Input: part model. Units: mm. Frame: model coordinates. Round coordinates to 2 decimals unless told otherwise and drop trailing zeros. Order: outer loops, then holes, each group sorted by start corner. A loop starts at its lowest first (then second) coordinate and runs counter-clockwise, first axis right, second up.
Item 1: Cut plane B-B on x = -10. Output: boundary loops of the cut face in (y, z).
Item 2: Line query: L1, parallel to Y at x = 0, z = -18.5; L2, parallel to Z at x = 2, y = -429.5 (3 decimals); L3, parallel to X at y = -786, z = 0.5. Output: solid intervals per line, ascending.
Item 3: Cut plane A-A on z = 0. Output: boundary loops of the cut face in (x, y), then the cut area to 3 significant figures.
Item 4: Cut plane C-C on y = -773. Output: boundary loops of the cut face in (x, z), then the cut area to 3 significant figures.
Item 5: First-contact query: pin 1 (5 mm diameter, centred on y = -100.5, z = -13.5, fed in from +X); pin 2 (6 mm diameter, centred on y = -367, z = 3.5, fed in from -X); pin 3 (4 mm diameter, centred on x = 11.5, y = -325.5, fed in from +Z). Flat tips, straight axial feed; report the tip coordinate or a pass-through.
```python
from build123d import *

# Parameters (mm, degrees)
F0_R     = 19.05
F0_R_2   = 17.45
F1_DEPTH = 825
F2_R     = 3.5625283299
F3_DEPTH = 20.050000094
F4_R     = 1
F5_DEPTH = 20.050000107


with BuildPart() as f1:
    # F0 (on Front) → F1 (new body)
    with BuildSketch(Plane.XZ):
        Circle(F0_R)
        Circle(F0_R_2, mode=Mode.SUBTRACT)
    extrude(amount=F1_DEPTH)

    # F2 (on Top) → F3 (cut, up to face)
    with BuildSketch(Plane.XY):
        with Locations((0, -140)):
            Circle(F2_R)
    extrude(amount=F3_DEPTH, mode=Mode.SUBTRACT)

    # F4 (on Top) → F5 (cut, up to face)
    with BuildSketch(Plane.XY):
        with Locations((0, -15)):
            Circle(F4_R)
    extrude(amount=-F5_DEPTH, mode=Mode.SUBTRACT)


solid = f1.part
```
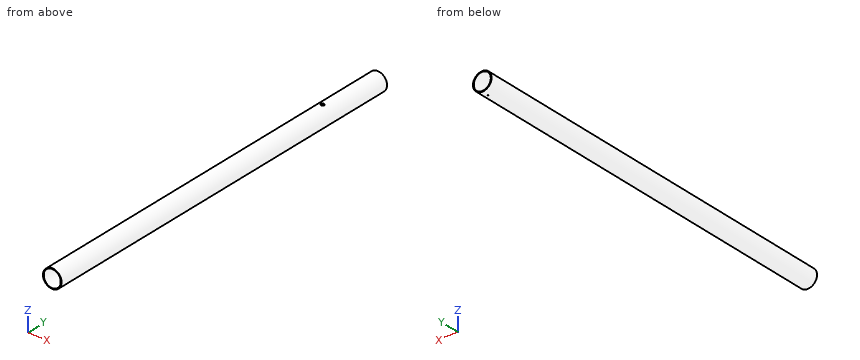
From the geometry:
1. outline: (-825, -16.21) - (0, -16.21) - (0, -14.3) - (-825, -14.3) - close; (-825, 14.3) - (0, 14.3) - (0, 16.21) - (-825, 16.21) - close
2. L1: y = -825 to -16, -14 to 0
2. L2: z = -18.945 to -17.335, 17.335 to 18.945
2. L3: x = -19.04 to -17.44, 17.44 to 19.04
3. outline: (-19.05, -825) - (-17.45, -825) - (-17.45, 0) - (-19.05, 0) - close; (17.45, -825) - (19.05, -825) - (19.05, 0) - (17.45, 0) - close
3. area: 2,640 mm2
4. outline: circle Ø38.1 at (0, 0); hole circle Ø34.9 at (0, 0)
4. area: 183 mm2
5. pin 1: stops at x = 15.55
5. pin 2: stops at x = -19.04
5. pin 3: stops at z = 16.51
